Can you work these out from the model? Positions are in its coordinate system, mm. Round coordinates to 2 decimals unless told otherwise and drop trailing zeros. Write each loop counter-clockwise with the first axis right and the second up, starting at its lowest first coordinate (ties: lowest second). Pieces come first, ordered by that corner, then holes. Notation, with made-up numbers: M 21,69.25 L 45,69.25 A22 ccw 45,85.25 Z; hole C -24,70 d2. An arc over 180 degrees is marked long. Answer in a Markdown table with one row per item. Add a question column.
(1) Suppose I cut it at B-B, the plane z = -700. Write out the boundary of the cut face in (x, y).
(2) Suppose I cut it at C-C, the plane x = 700. Write out the boundary of the cut face in (y, z).
(3) If we mould it in two halves opening along Z, with no side actions, what happens to faces 1 (the face through (696, 200, -704)), 2 (the face through (1400, 296, -690)), 3 (the face through (710, 296, -1400)), 4 (the face through (938.455, 402.8, -775.093))? For each: released by +Z, released by -Z, zero draft, split by the parting line, or undercut.
(4) If I drill on probe 1 along Z at (x, y) = (700, 436); probe 2 along X at (y, z) = (392, -700); probe 3 along Y at (x, z) = (552, -529.5), over which ranges is the centre line in solid material (lowest first)?
(5) Suppose I cut it at A-A, the plane y = 300.5. Write out the boundary of the cut face in (x, z), then the cut area to 3 significant figures.
(6) I'm going to push a flat-ended pin straight in: pin 1 (12 mm diameter, centred on x = 760, z = -1039, fed in from -Y). Where does the tip first touch, or does it pass through?
Autodesk Inventor part; units mm, degrees
ref_plane "YZ Plane" through (0, 0, 0) normal (1, 0, 0) x (0, 1, 0)
ref_plane "XZ Plane" through (0, 0, 0) normal (0, 1, 0) x (-1, 0, 0)
ref_plane "XY Plane" through (0, 0, 0) normal (0, 0, 1) x (1, 0, 0)
sketch "Boceto1" plane through (0, 0, 0) normal (0, 1, 0) x (-1, 0, 0)
  line L0 (0, 0) -> (-1400, 0)
  line L1 (-1400, 0) -> (-1400, -1400)
  line L2 (-1400, -1400) -> (0, -1400)
  line L3 (0, -1400) -> (0, 0)
  dimension "d0" = 1400
  dimension "d1" = 1400
extrude "Extrusión1" add sketch "Boceto1" along normal blind 600
sketch "Boceto2" plane through (0, 600, 0) normal (0, 1, 0) x (1, 0, 0)
  line L0 (0, 0) -> (800, 0)
  circle A0 centre (700, 700) radius 250
  line L1 (0, 1400) -> (0, 0)
  line L2 (1400, 1400) -> (0, 1400)
  dimension "d6" = 500
  dimension "d9" = 700
  dimension "d10" = 700
extrude "Extrusión2" cut sketch "Boceto2" against normal blind 400
properties part number "Soporte"
Calculated:
| question | item | result |
|---|---|---|
| 1 | outline | M 0,0 L 1400,0 L 1400,600 L 950,600 L 950,200 L 450,200 L 450,600 L 0,600 Z |
| 2 | outline | M 0,-1400 L 600,-1400 L 600,-950 L 200,-950 L 200,-450 L 600,-450 L 600,0 L 0,0 Z |
| 3 | face 1 | undercut |
| 3 | face 2 | zero draft |
| 3 | face 3 | released by -Z |
| 3 | face 4 | undercut |
| 4 | probe 1 | -1400 to -950, -450 to 0 |
| 4 | probe 2 | 0 to 450, 950 to 1400 |
| 4 | probe 3 | 0 to 200 |
| 5 | outline | M 0,-1400 L 1400,-1400 L 1400,0 L 0,0 Z; hole C 700,-700 d500 |
| 5 | area | 1,760,000 mm² |
| 6 | pin 1 | y = 0 |
